Geometry: see drawing. Coordinates: mm, zero at the bounding-box minimum. A direction names the side the tool comes from. Give positions to 0.01 mm unless a question says otherwise; leave off trailing zeros. Order: outer loops, then holes, each group sorted by start corner. A loop starts at its lowest first (then second) coordinate and runs counter-clockwise, first axis right, second up. Notation, with made-up numbers: (89.25, 9.25) -> (145.25, 9.25) arc R20 cw to (145.25, 26.25) -> close; hole circle Ø6 at (28, -9). An arc over 180 degrees is marked (long way). One line per item, written item: value. Start each with the question number.
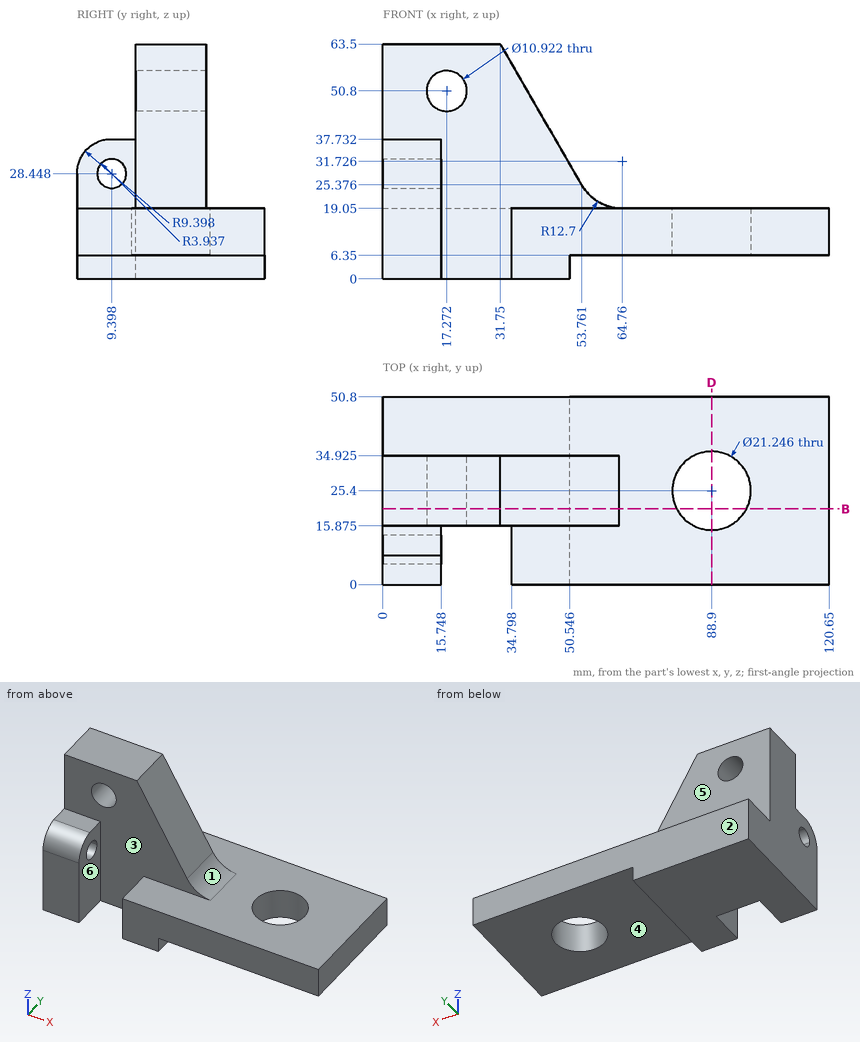
1. Cut plane B-B, the plane y = 20.5. State how many separate pieces and enclosed holes the cut face has, then the cut area to 3 significant figures.
2. Material intervals for L1, parallel to Y at x = 88.9, z = 9.25; L2, parallel to Y at x = 30, z = 28.5 (1 decimal); L3, parallel to Z at x = 67, y = 22.5, sorted ascending. Write a range as [from, to].
3. Pin query (flat end, axial travel): P1, Ø5, axis at y = 9, z = 24.5, coming from the -X side; P2, Ø14, axis at x = 17.272, z = 50.8, coming from the +Y side (3 decimals); P3, Ø10, axis at y = 23, z = 29.5, coming from the +X side (1 decimal); P4, Ø1, axis at x = 58.5, y = 33.5, coming from the -Z side. Return the tip coordinate at first contact, or that it passes through.
4. Access query for the marked faces 4, 5 and 6. Directions: +Z, -Z, +X, -X, +Y, -Y. A direction counts if a zero-diameter tool reaches every point of the face in a straight line with its end or side. Return the directions, or none.
5. Cut plane D-D, the plane x = 88.9. Return loops of the section in (y, z).
6. Draft query along X for the marked faces 1, 2 and 3. Return one class per face: pulls with the +X half, pulls with the -X half, needs draft (parallel to the pull), parting line crosses it, or undercut.
Answers follow:
1. separate pieces: 2
1. enclosed holes: 1
1. area: 3,510 mm²
2. L1: y = [0, 14.78], [36.02, 50.8]
2. L2: y = [15.9, 34.9]
2. L3: z = [6.35, 19.05]
3. P1: stops at x = 0
3. P2: stops at y = 34.925
3. P3: stops at x = 54.3
3. P4: stops at z = 6.35
4. face 4: -Z, +X, +Y, -Y
4. face 5: +Z, +X, -X, +Y
4. face 6: +Z, -Z, -Y
5. outline: (0, 6.35) -> (14.78, 6.35) -> (14.78, 19.05) -> (0, 19.05) -> close; (36.02, 6.35) -> (50.8, 6.35) -> (50.8, 19.05) -> (36.02, 19.05) -> close
6. face 1: pulls with the +X half
6. face 2: needs draft
6. face 3: undercut
